Verification items for the finished model (mm, model axes). Face numbers are marked on the shaded views. A direction names the side the tool comes from. Round coordinates to 2 decimals unless told otherwise and drop trailing zeros. Order: outer loops, then holes, each group sorted by start corner. A loop starts at its lowest first (then second) coordinate and runs counter-clockwise, first axis right, second up. Notation, with made-up numbers: M 26.25,65 L 59.25,65 A28 ccw 59.25,99 Z; hole C 16,63 d10. An arc over 180 degrees is marked long. Return JSON: item names as keys, results as strings. Group by question number.
from build123d import *

# Parameters (mm, degrees)
BOSS_EXTRUDE2_DEPTH              = 4.7625
SKETCH3_W                        = 3.175
SKETCH3_H                        = 9.525
CUT_EXTRUDE1_DEPTH               = 10.16
SKETCH4_W                        = 9.525
SKETCH4_H                        = 9.525
BOSS_EXTRUDE3_DEPTH              = 6.35
F_8_32_TAPPED_HOLE1_D            = 3.4544
F_8_32_TAPPED_HOLE1_DEPTH        = 9.525
F_8_32_TAPPED_HOLE1_TIP          = 1.037806461
F_1_8_0_125_DIAMETER_HOLE1_D     = 3.175
F_1_8_0_125_DIAMETER_HOLE1_DEPTH = 3.175
F_4_40_TAPPED_HOLE1_D            = 2.2606


with BuildPart() as part:
    # Sketch2 → Boss-Extrude2 (new body, symmetric)
    with BuildSketch(Plane.XY):
        with BuildLine():
            Line((-9.525, 4.7625), (0, 4.7625))
            ThreePointArc((0, 4.7625), (4.7625, 0), (0, -4.7625))
            Line((0, -4.7625), (-9.525, -4.7625))
            Line((-9.525, -4.7625), (-9.525, 4.7625))
        make_face()
    extrude(amount=BOSS_EXTRUDE2_DEPTH, both=True)

    # Sketch3 → Cut-Extrude1 (cut)
    with BuildSketch(Plane(origin=(4.7625, 0, 0), x_dir=(0, 0, -1), z_dir=(1, 0, 0))):
        Rectangle(SKETCH3_W, SKETCH3_H)
    extrude(amount=-CUT_EXTRUDE1_DEPTH, mode=Mode.SUBTRACT)

    # Sketch4 → Boss-Extrude3 (add)
    with BuildSketch(Plane.ZY.offset(9.525)):
        Rectangle(SKETCH4_W, SKETCH4_H)
    extrude(amount=BOSS_EXTRUDE3_DEPTH)

    # #8-32 Tapped Hole1
    with Locations(Plane.ZY.offset(15.875)):
        with Locations((0, 0)):
            Hole(F_8_32_TAPPED_HOLE1_D / 2, depth=F_8_32_TAPPED_HOLE1_DEPTH)
            with Locations((0, 0, -(F_8_32_TAPPED_HOLE1_DEPTH + F_8_32_TAPPED_HOLE1_TIP / 2))):  # 118° drill point
                Cone(0, F_8_32_TAPPED_HOLE1_D / 2, F_8_32_TAPPED_HOLE1_TIP, mode=Mode.SUBTRACT)

    # 1/8 (0.125) Diameter Hole1
    with Locations(Plane.XY.offset(4.7625)):
        with Locations((0, 0)):
            Hole(F_1_8_0_125_DIAMETER_HOLE1_D / 2, depth=F_1_8_0_125_DIAMETER_HOLE1_DEPTH)

    # #4-40 Tapped Hole1 (through all)
    with Locations(Plane.XY.offset(-1.5875)):
        with Locations((0, 0)):
            Hole(F_4_40_TAPPED_HOLE1_D / 2)


solid = part.part
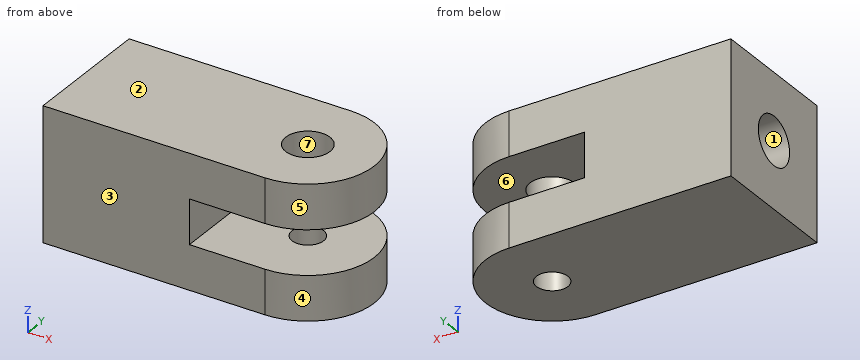
1. Draft check along Y on the marked faces 1, 2, 3 and 4. Enter one of: +Y half, -Y half, draft (parallel to the pull), parting line (faces both ways), or undercut.
2. Cross-section at C-C (y = 0). Give the number of separate pieces and of enclosed holes in the cut face, plus the area to 3 significant figures.
3. Cross-section at D-D (x = -0.5). Enter the section's corners in (y, z), plus the area to 3 significant figures.
4. Thickness scan on line 1 along Z through (x, y) = (-4.5, -3); line 2 along Y through (x, z) = (-11.75, 0). Record the ranges inside material, lowest first. Write a range as from..to.
5. Go/stop test with flat-tipped pins: pin 1 (3 mm diameter, centred on y = 0, z = 0, fed in from +X); pin 2 (1 mm diameter, centred on y = 1, z = 2, fed in from +X); pin 3 (1.5 mm diameter, centred on y = 1, z = 1.5, fed in from +X). Record where each tip stops, or that it passes through.
6. Access from +Z, -Z, +X, -X, +Y, -Y to the whole of each face (thin tool, end or side, straight path). Record for the marked faces 5, 6 and 7.
7. Cross-section at B-B (x = -10.5). Enter the section's corners in (y, z).
8. Cross-section at A-A (z = -2.75). Enter the section's corners in (x, y) (1 decimal), plus the area to 3 significant figures.
Computed:
{
 "1": {"face 1": "undercut", "face 2": "draft", "face 3": "-Y half", "face 4": "parting line"},
 "2": {"separate pieces": "4", "enclosed holes": "0", "area": "112 mm²"},
 "3": {"outline": "M -4.76,-4.76 L -1.01,-4.76 L -1.01,-1.59 L -4.76,-1.59 Z; M -4.76,1.59 L -1.51,1.59 L -1.51,4.76 L -4.76,4.76 Z; M 1.01,-4.76 L 4.76,-4.76 L 4.76,-1.59 L 1.01,-1.59 Z; M 1.51,1.59 L 4.76,1.59 L 4.76,4.76 L 1.51,4.76 Z", "area": "44.5 mm²"},
 "4": {"line 1": "z = -4.76..-1.59, 1.59..4.76", "line 2": "y = -4.76..-1.73, 1.73..4.76"},
 "5": {"pin 1": "stops at x = -5.4", "pin 2": "stops at x = 4.74", "pin 3": "stops at x = 4.76"},
 "6": {"face 5": "+Z, -Z, +X", "face 6": "+X, +Y, -Y", "face 7": "+Z"},
 "7": {"outline": "M -4.76,-4.76 L 4.76,-4.76 L 4.76,4.76 L -4.76,4.76 Z; hole C 0,0 d3.45"},
 "8": {"outline": "M -15.9,-4.8 L 0,-4.8 A4.8 ccw 0,4.8 L -15.9,4.8 Z; hole C 0,0 d2.3", "area": "183 mm²"}
}
